Model file for the job. Use its own axes, mm. A direction names the side the tool comes from. Give positions to 0.01 mm unless a question says otherwise; leave off trailing zeros. Loops run counter-clockwise (first coordinate to the right, second up) from the corner with the lowest first, then second, coordinate; pieces in that order, holes last. Notation, with made-up numbers: (73, 82) - (104, 82) arc R14 ccw to (104, 88) - close; hole circle Ø8 at (18.5, -10.5). An arc over 180 degrees is marked (long way). Use a Markdown table: item, result.
from build123d import *

# Parameters (mm, degrees)
BOSS_EXTRU_1_DEPTH       = 24
CONG_1_R                 = 3
ESQUISSE2_R              = 4.25
ENL_V_MAT_EXTRU_1_DEPTH  = 110.65086639
ESQUISSE3_R              = 4.25
ENL_V_MAT_EXTRU_2_DEPTH  = 94.22236856
ESQUISSE4_R              = 3.25
ENL_V_MAT_EXTRU_3_DEPTH  = 1.5
ENL_V_MAT_EXTRU_4_DEPTH  = 99.696010558
CONG_2_R                 = 1
ESQUISSE7_R              = 3.25
BOSS_EXTRU_2_DEPTH       = 3
ESQUISSE8_R              = 7.55
ENL_V_MAT_EXTRU_7_DEPTH  = 1.1
ESQUISSE9_R              = 6.55
ENL_V_MAT_EXTRU_8_DEPTH  = 5
ENL_V_MAT_EXTRU_13_DEPTH = 94.22236856


with BuildPart() as part:
    # Esquisse1 → Boss.-Extru.1 (new body)
    with BuildSketch(Plane.XY):
        Polygon((-25.05, 0), (25.05, 0), (25.05, 22), (-25.05, 22), (-25.05, 54), (-79.05, 54), (-79.05, 0), (-47.05, 0), (-47.05, -50.1), (-25.05, -50.1), align=None)
    extrude(amount=-BOSS_EXTRU_1_DEPTH)

    # Cong_1
    cong_1_edges = [part.edges().sort_by_distance(p)[0] for p in [
        (-25.05, 0, -12),
    ]]
    fillet(cong_1_edges, radius=CONG_1_R)

    # Esquisse2 → Enl_v. mat.-Extru.1 (cut, through all)
    with BuildSketch(Plane(origin=(0, 22, 0), x_dir=(1, 0, 0), z_dir=(0, 1, 0))):
        with Locations(Location((0, 12, 0), (0, 0, 270))):
            Circle(ESQUISSE2_R)
    extrude(amount=-ENL_V_MAT_EXTRU_1_DEPTH, mode=Mode.SUBTRACT)

    # Esquisse3 → Enl_v. mat.-Extru.2 (cut, through all)
    with BuildSketch(Plane.ZY.offset(47.05)):
        with Locations(Location((-12, -25.05, 0), (0, 0, 270))):
            Circle(ESQUISSE3_R)
    extrude(amount=-ENL_V_MAT_EXTRU_2_DEPTH, mode=Mode.SUBTRACT)

    # Esquisse4 → Enl_v. mat.-Extru.3 (cut)
    with BuildSketch(Plane.XY):
        with BuildLine():
            Line((-67.05, 47.6), (-67.05, 21.4))
            ThreePointArc((-67.05, 21.4), (-52.05, 6.4), (-37.05, 21.4))
            Line((-37.05, 21.4), (-37.05, 47.6))
            Line((-37.05, 47.6), (-67.05, 47.6))
        make_face()
        with Locations((-52.05, 21.4)):
            Circle(ESQUISSE4_R, mode=Mode.SUBTRACT)
    extrude(amount=-ENL_V_MAT_EXTRU_3_DEPTH, mode=Mode.SUBTRACT)

    # Esquisse4_2 → Enl_v. mat.-Extru.4 (cut, through all)
    with BuildSketch(Plane.XY):
        with BuildLine():
            ThreePointArc((-48.8, 21.4), (-52.05, 24.65), (-55.3, 21.4))
            Line((-55.3, 21.4), (-48.8, 21.4))
        make_face()
        with BuildLine():
            Line((-48.8, 21.4), (-55.3, 21.4))
            ThreePointArc((-55.3, 21.4), (-52.05, 18.15), (-48.8, 21.4))
        make_face()
    extrude(amount=-ENL_V_MAT_EXTRU_4_DEPTH, mode=Mode.SUBTRACT)

    # Cong_2
    cong_2_edges = [part.edges().sort_by_distance(p)[0] for p in [
        (-47.05, -25.05, -24),
        (-79.05, 27, 0),
        (-52.05, 54, 0),
        (-25.05, 38, 0),
        (0, 22, 0),
        (25.05, 11, 0),
        (-36.05, -50.1, 0),
        (-47.05, -25.05, 0),
        (-36.05, -50.1, -24),
        (-63.05, 0, 0),
        (-79.05, 0, -12),
        (-79.05, 54, -12),
        (-25.05, 54, -12),
        (-25.05, 22, -12),
        (25.05, 22, -12),
        (25.05, 0, -12),
        (-25.05, -50.1, -12),
        (-47.05, -50.1, -12),
        (-47.05, 0, -12),
        (25.05, 11, -24),
        (-25.05, -26.55, 0),
        (-25.05, -26.55, -24),
        (1.5, 0, 0),
        (1.5, 0, -24),
        (-24.171320344, -0.878679656, 0),
        (-24.171320344, -0.878679656, -24),
        (0, 22, -24),
        (-25.05, 38, -24),
        (-52.05, 54, -24),
        (-79.05, 27, -24),
        (-63.05, 0, -24),
    ]]
    fillet(cong_2_edges, radius=CONG_2_R)

    # Esquisse7 → Boss.-Extru.2 (add)
    with BuildSketch(Plane.XY):
        with BuildLine():
            Line((-67.05, 47.6), (-37.05, 47.6))
            Line((-37.05, 47.6), (-37.05, 21.4))
            ThreePointArc((-37.05, 21.4), (-52.05, 6.4), (-67.05, 21.4))
            Line((-67.05, 21.4), (-67.05, 47.6))
        make_face()
        with Locations((-52.05, 21.4)):
            Circle(ESQUISSE7_R, mode=Mode.SUBTRACT)
    extrude(amount=-BOSS_EXTRU_2_DEPTH)

    # Esquisse8 → Enl_v. mat.-Extru.7 (cut)
    with BuildSketch(Plane.XY):
        with Locations((-52.05, 21.4)):
            Circle(ESQUISSE8_R)
    extrude(amount=-ENL_V_MAT_EXTRU_7_DEPTH, mode=Mode.SUBTRACT)

    # Esquisse9 → Enl_v. mat.-Extru.8 (cut)
    with BuildSketch(Plane.XY):
        with Locations((-52.05, 21.4)):
            Circle(ESQUISSE9_R)
    extrude(amount=-ENL_V_MAT_EXTRU_8_DEPTH, mode=Mode.SUBTRACT)

    # Esquisse14 → Enl_v. mat.-Extru.13 (cut, through all)
    with BuildSketch(Plane.ZY.offset(47.05)):
        with BuildLine():
            Line((-16.25, -25.05), (-16.25, -50.1))
            Line((-16.25, -50.1), (-7.75, -50.1))
            Line((-7.75, -50.1), (-7.75, -25.05))
            ThreePointArc((-7.75, -25.05), (-12, -20.8), (-16.25, -25.05))
        make_face()
    extrude(amount=-ENL_V_MAT_EXTRU_13_DEPTH, mode=Mode.SUBTRACT)


solid = part.part
(1) Slice it at B-B, the plane x = -52.05. Write the cut outline in (y, z), plus the area to 3 significant figures.
Computed:
| item | result |
|---|---|
| outline | (0, -23) arc R1 ccw to (1, -24) - (18.15, -24) - (18.15, -5) - (14.85, -5) - (14.85, -1.1) - (13.85, -1.1) - (13.85, 0) - (1, 0) arc R1 ccw to (0, -1) - close; (24.65, -24) - (53, -24) arc R1 ccw to (54, -23) - (54, -1) arc R1 ccw to (53, 0) - (28.95, 0) - (28.95, -1.1) - (27.95, -1.1) - (27.95, -5) - (24.65, -5) - close |
| area | 1,100 mm² |
(2) Slice it at C-C, the plane y = -33. Write the cut outline in (x, z), plus the area to 3 significant figures.
Computed:
| item | result |
|---|---|
| outline | (-47.05, -23) arc R1 ccw to (-46.05, -24) - (-26.05, -24) arc R1 ccw to (-25.05, -23) - (-25.05, -16.25) - (-47.05, -16.25) - close; (-47.05, -7.75) - (-25.05, -7.75) - (-25.05, -1) arc R1 ccw to (-26.05, 0) - (-46.05, 0) arc R1 ccw to (-47.05, -1) - close |
| area | 340 mm² |
(3) 3-axis set-ups, long thin cutter, end or side, ignore diameter. For faces 4 (the flat face through (-63, 0, -12)), 5 (the flat face through (-25.05, 38, -12)), 6 (the flat face through (-36, -37, -16.25)), 7 (the cylindrical face through (-46, 18.89, -3.02)): which of +Z, -Z, +X, -X, +Y, -Y reach the whole face in a straight line?
Computed:
| item | result |
|---|---|
| face 4 | +Z, -Z, -X, -Y |
| face 5 | +Z, -Z, +X, +Y |
| face 6 | +X, -X, -Y |
| face 7 | +Z |
(4) Mould opens along Z. For faces 1 (the flat face through (-52, 54, -12)), 2 (the cylindrical face through (1.277, 11.154, -7.946)), 3 (the flat face through (-49, 19, -5)) say: pulls with the +Z half, pulls with the -Z half, needs draft (parallel to the pull), parting line crosses it, or undercut.
Computed:
| item | result |
|---|---|
| face 1 | needs draft |
| face 2 | undercut |
| face 3 | pulls with the +Z half |
(5) Pin check, flat tips, straight feed: P1, Ø2, axis at y = -3.5, z = -5, coming from the +X side; P2, Ø12, axis at y = -13.5, z = -10, coming from the +X side; P3, Ø15, axis at x = -52.05, y = 21.4, coming from the +Z side. Stop position of each tip, or through.
Computed:
| item | result |
|---|---|
| P1 | x = -25.01 |
| P2 | x = -25.05 |
| P3 | z = -1.1 |
(6) Slice it at A-A, the plane z = -12. Write the cut outline in (x, y).
Computed:
| item | result |
|---|---|
| outline | (-79.05, 1) arc R1 ccw to (-78.05, 0) - (-48.05, 0) arc R1 cw to (-47.05, -1) - (-47.05, -20.8) - (-25.05, -20.8) - (-25.05, -3) arc R3 cw to (-22.05, 0) - (-4.25, 0) - (-4.25, 22) - (-24.05, 22) arc R1 cw to (-25.05, 23) - (-25.05, 53) arc R1 ccw to (-26.05, 54) - (-78.05, 54) arc R1 ccw to (-79.05, 53) - close; (4.25, 0) - (24.05, 0) arc R1 ccw to (25.05, 1) - (25.05, 21) arc R1 ccw to (24.05, 22) - (4.25, 22) - close; hole circle Ø6.5 at (-52.05, 21.4) |
(7) Drill centre lines: probe 1 along Z at (x, y) = (-29.5, -42); probe 2 along Y at (x, z) = (-52.05, -3.95); probe 3 along Y at (x, z) = (-52.05, -18). Where is each one in solid material? Low to high. Write a range as [from, to].
Computed:
| item | result |
|---|---|
| probe 1 | [-24, -16.25], [-7.75, 0] |
| probe 2 | [0, 14.85], [27.95, 54] |
| probe 3 | [0, 18.15], [24.65, 54] |
(8) Slice it at D-D, the plane z = -6.5. Write the cut outline in (x, y), plus the area to 3 significant figures.
Computed:
| item | result |
|---|---|
| outline | (-79.05, 1) arc R1 ccw to (-78.05, 0) - (-48.05, 0) arc R1 cw to (-47.05, -1) - (-47.05, -49.1) arc R1 ccw to (-46.05, -50.1) - (-26.05, -50.1) arc R1 ccw to (-25.05, -49.1) - (-25.05, -3) arc R3 cw to (-22.05, 0) - (24.05, 0) arc R1 ccw to (25.05, 1) - (25.05, 21) arc R1 ccw to (24.05, 22) - (-24.05, 22) arc R1 cw to (-25.05, 23) - (-25.05, 53) arc R1 ccw to (-26.05, 54) - (-78.05, 54) arc R1 ccw to (-79.05, 53) - close; hole circle Ø6.5 at (-52.05, 21.4) |
| area | 5,090 mm² |
